Verification items for the finished model (mm, model axes). Face numbers are marked on the shaded views. A direction names the side the tool comes from. Round coordinates to 2 decimals unless told otherwise and drop trailing zeros. Loops run counter-clockwise (first coordinate to the right, second up) from the corner with the lowest first, then second, coordinate; pieces in that order, holes last. Notation, with made-up numbers: M -0.5,53.25 L 37.5,53.25 A23 ccw 37.5,89.25 Z; hole C 13,14 d4. An arc over 180 degrees is marked long. Write item = value, one per line. Start each with the question number.
from build123d import *

# Parameters (mm, degrees)
SKETCH_1_R          = 5
EXTRUDE_1_DEPTH     = 3
SKETCH_2_R          = 1.5
CUT_EXTRUDE_1_DEPTH = 11
SKETCH_3_R          = 5
SKETCH_3_R_2        = 4
CUT_EXTRUDE_3_DEPTH = 0.5


with BuildPart() as part:
    # 草图1 → 凸台-拉伸1 (new body)
    with BuildSketch(Plane(origin=(0, 0, 0), x_dir=(1, 0, 0), z_dir=(0, 1, 0))):
        Circle(SKETCH_1_R)
    extrude(amount=EXTRUDE_1_DEPTH)

    # 草图2 → 切除-拉伸1 (cut)
    with BuildSketch(Plane(origin=(0, 3, 0), x_dir=(1, 0, 0), z_dir=(0, 1, 0))):
        Circle(SKETCH_2_R)
    extrude(amount=-CUT_EXTRUDE_1_DEPTH, mode=Mode.SUBTRACT)

    # 草图3 → 切除-拉伸3 (cut, symmetric)
    with BuildSketch(Plane(origin=(0, 1.5, 0), x_dir=(-1, 0, 0), z_dir=(0, -1, 0))):
        Circle(SKETCH_3_R)
        Circle(SKETCH_3_R_2, mode=Mode.SUBTRACT)
    extrude(amount=CUT_EXTRUDE_3_DEPTH, both=True, mode=Mode.SUBTRACT)


solid = part.part
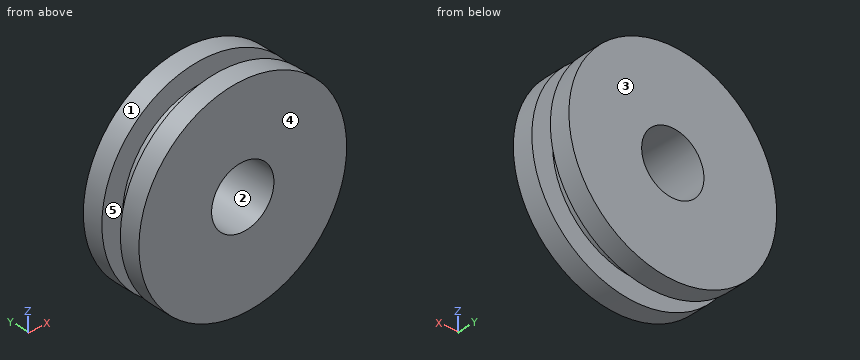
1. Section check A-A, the plane x = 0. Enter the section's corners in (y, z), and give its area (3 significant figures).
2. Section check C-C, the plane y = 1.35. Enter the section's corners in (x, z), and give its area (3 significant figures).
3. Mould release check, pull along Z, two halves, no side actions. Record for the marked faces 1, 2 and 3: pulls with the +Z half, pulls with the -Z half, needs draft (parallel to the pull), parting line crosses it, or undercut.
4. Thickness scan on line 1 (Y direction, x = -0.5, z = -4.25); line 2 (Z direction, x = 0, y = 1.05). Record the ranges inside material, lowest first.
5. Tool access check on the marked faces 4 and 5. Record the directions out of +Z, -Z, +X, -X, +Y, -Y that give a thin tool (end or side, any length) a straight path to the whole face; none if there is none.
6. Gauge pin test, flat ends, axial feed: P1, Ø1, axis at y = 1, z = 1, coming from the -X side; P2, Ø6, axis at x = -1, z = 1.5, coming from the -Y side; P3, Ø1.5, axis at y = 2, z = 2, coming from the +X side; P4, Ø1.5, axis at y = 0.5, z = -3, coming from the -X side. Record the tip position at first contact, or that the pin passes through.
7. Section check B-B, the plane z = 0. Enter the section's corners in (x, y).
8. Section check D-D, the plane z = 2. Enter the section's corners in (x, y).
Computed values:
q1.outline = M 0,-5 L 1,-5 L 1,-4 L 2,-4 L 2,-5 L 3,-5 L 3,-1.5 L 0,-1.5 Z; M 0,1.5 L 3,1.5 L 3,5 L 2,5 L 2,4 L 1,4 L 1,5 L 0,5 Z
q1.area = 19.0 mm2
q2.outline = C 0,0 d8; hole C 0,0 d3
q2.area = 43.2 mm2
q3.face_1 = parting line crosses it
q3.face_2 = undercut
q3.face_3 = needs draft
q4.line_1 = 0 to 1, 2 to 3
q4.line_2 = -4 to -1.5, 1.5 to 4
q5.face_4 = +Z, -Z, +X, -X, -Y
q5.face_5 = none
q6.P1 = -4.97
q6.P2 = 0
q6.P3 = 4.84
q6.P4 = -4.47
q7.outline = M -5,0 L -1.5,0 L -1.5,3 L -5,3 L -5,2 L -4,2 L -4,1 L -5,1 Z; M 1.5,0 L 5,0 L 5,1 L 4,1 L 4,2 L 5,2 L 5,3 L 1.5,3 Z
q8.outline = M -4.58,0 L 4.58,0 L 4.58,1 L 3.46,1 L 3.46,2 L 4.58,2 L 4.58,3 L -4.58,3 L -4.58,2 L -3.46,2 L -3.46,1 L -4.58,1 Z
